Model file for the job. Use its own axes, mm. Coordinates: 2 decimals unless noted, no trailing zeros. Order: outer loops, then holes, each group sorted by start corner. A loop starts at its lowest first (then second) coordinate and runs counter-clockwise, first axis right, second up. Notation, with made-up numbers: (47, 58) -> (53, 58) arc R12 ccw to (53, 71) -> close; hole circle Ø6 at (75.25, 55). An arc over 180 degrees is marked (long way). Return JSON: item names as keys, results as strings. Group by question number.
1) Probe line 1 (X direction, y = 23, z = 22); line 2 (Z direction, x = -50, y = 27); line 3 (Y direction, x = -18.5, z = 57). List the from-to ranges inside material, lowest first.
2) Cut at C-C (x = 22). Write the cut outline in (y, z).
3) Cut at B-B (z = 15). Write the cut outline in (x, y).
4) Cut at A-A (y = 6). Write the cut outline in (x, z).
5) Flat gauge pins, fed straight in: pin 1 (3.5 mm diameter, centred on x = -50.5, y = 21.5, fed in from +Z); pin 2 (2.5 mm diameter, centred on y = 24.5, z = -16, fed in from +X); pin 3 (1.5 mm diameter, centred on y = 14.5, z = 62, fed in from -X). Where does each tip first touch, or does it go through?
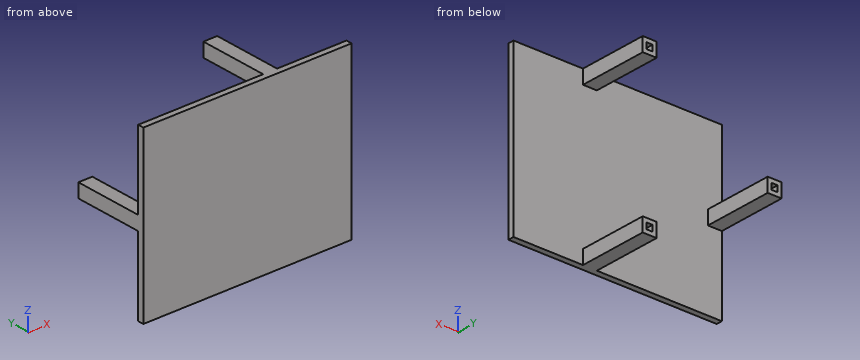
from build123d import *

# Parameters (mm, degrees)
SKETCH3_W           = 105
SKETCH3_H           = 85
BOSS_EXTRUDE3_DEPTH = 3
SKETCH5_W           = 7
SKETCH5_H           = 7
SKETCH5_W_2         = 3
SKETCH5_H_2         = 3
BOSS_EXTRUDE4_DEPTH = 35
SKETCH9_W           = 2.998895248
SKETCH9_H           = 2.995380601
BOSS_EXTRUDE5_DEPTH = 35
SKETCH11_W          = 7
SKETCH11_H          = 7
SKETCH11_W_2        = 3
SKETCH11_H_2        = 3
BOSS_EXTRUDE6_DEPTH = 35


with BuildPart() as part:
    # Sketch3 → Boss-Extrude3 (new body)
    with BuildSketch(Plane(origin=(0, 0, 0), x_dir=(1, 0, 0), z_dir=(0, 1, 0))):
        with Locations((-2.316884661, -22.898810939)):
            Rectangle(SKETCH3_W, SKETCH3_H)
    extrude(amount=BOSS_EXTRUDE3_DEPTH)

    # Sketch5 → Boss-Extrude4 (add)
    with BuildSketch(Plane(origin=(0, 3, 0), x_dir=(1, 0, 0), z_dir=(0, 1, 0))):
        with Locations((11.683115339, -61.898810939)):
            Rectangle(SKETCH5_W, SKETCH5_H)
        with Locations((11.683115339, -61.898810939)):
            Rectangle(SKETCH5_W_2, SKETCH5_H_2, mode=Mode.SUBTRACT)
    extrude(amount=BOSS_EXTRUDE4_DEPTH)

    # Sketch9 → Boss-Extrude5 (add)
    with BuildSketch(Plane(origin=(0, 3, 0), x_dir=(1, 0, 0), z_dir=(0, 1, 0))):
        Polygon((15.183115339, 12.601189061), (15.183115339, 19.601189061), (8.183115339, 19.601189061), (8.183115339, 17.600348451), (8.183115339, 12.601189061), align=None)
        with Locations((11.687877227, 16.102658151)):
            Rectangle(SKETCH9_W, SKETCH9_H, mode=Mode.SUBTRACT)
    extrude(amount=BOSS_EXTRUDE5_DEPTH)

    # Sketch11 → Boss-Extrude6 (add)
    with BuildSketch(Plane(origin=(0, 3, 0), x_dir=(1, 0, 0), z_dir=(0, 1, 0))):
        with Locations((-51.316884661, -22.898810939)):
            Rectangle(SKETCH11_W, SKETCH11_H)
        with Locations((-51.316884661, -22.898810939)):
            Rectangle(SKETCH11_W_2, SKETCH11_H_2, mode=Mode.SUBTRACT)
    extrude(amount=BOSS_EXTRUDE6_DEPTH)


solid = part.part
Answers below:
{
 "1": {"line 1": "x = -54.82 to -52.82, -49.82 to -47.82", "line 2": "z = 19.4 to 21.4, 24.4 to 26.4", "line 3": "y = 0 to 3"},
 "2": {"outline": "(0, -19.6) -> (3, -19.6) -> (3, 65.4) -> (0, 65.4) -> close"},
 "3": {"outline": "(-54.82, 0) -> (50.18, 0) -> (50.18, 3) -> (-54.82, 3) -> close"},
 "4": {"outline": "(-54.82, 19.4) -> (-47.82, 19.4) -> (-47.82, 26.4) -> (-54.82, 26.4) -> close; (8.18, -19.6) -> (15.18, -19.6) -> (15.18, -12.6) -> (8.18, -12.6) -> close; (8.18, 58.4) -> (15.18, 58.4) -> (15.18, 65.4) -> (8.18, 65.4) -> close; hole (-52.82, 21.4) -> (-49.82, 21.4) -> (-49.82, 24.4) -> (-52.82, 24.4) -> close; hole (10.18, 60.4) -> (13.18, 60.4) -> (13.18, 63.4) -> (10.18, 63.4) -> close; hole (10.19, -17.6) -> (13.19, -17.6) -> (13.19, -14.6) -> (10.19, -14.6) -> close"},
 "5": {"pin 1": "stops at z = 26.4", "pin 2": "stops at x = 15.18", "pin 3": "stops at x = 8.18"}
}
